Part model, mm, in its own coordinate system. A direction names the side the tool comes from. Give positions to 0.01 mm unless a question says otherwise; leave off trailing zeros. Write each loop counter-clockwise with the first axis right and the second up, starting at its lowest first coordinate (ties: lowest second). Pieces come first, ordered by that corner, then holes. Notation, with made-up numbers: M -9,41.5 L 3,41.5 A16 cw 3,69.5 Z; hole C 6.5,74 d11. An arc over 180 degrees is marked long. Write item = value, one per line. Start each with the question number.
from build123d import *

# Parameters (mm, degrees)
SKETCH1_R                                       = 3.302
BOSS_EXTRUDE1_DEPTH                             = 6.35
SKETCH2_R                                       = 16.4211
BOSS_EXTRUDE3_DEPTH                             = 6.35
BOSS_EXTRUDE3_DEPTH_BACK                        = 3.175
F_6_CLEARANCE_HOLE1_D                           = 4.3053
F_6_CLEARANCE_HOLE1_DEPTH                       = 9.525
F_6_PLASTIC_INSERT_AT_2_COUNT                   = 2
F_6_PLASTIC_INSERT_AT_2_PITCH                   = 46.355
BOSS_EXTRUDE4_REACH                             = 14.7
SKETCH22_R                                      = 16.4211
SKETCH22_R_2                                    = 3.302
CBORE_FOR_0_PAN_HEAD_MACHINE_SCREW1_D           = 1.8542
CBORE_FOR_0_PAN_HEAD_MACHINE_SCREW1_CBORE_D     = 3.57124
CBORE_FOR_0_PAN_HEAD_MACHINE_SCREW1_CBORE_DEPTH = 6.35


with BuildPart() as part:
    # Sketch1 → Boss-Extrude1 (new body)
    with BuildSketch(Plane.XY):
        with BuildLine():
            ThreePointArc((16.170566439, -2.8575), (16.4211, 0), (16.170566439, 2.8575))
            ThreePointArc((16.170566439, 2.8575), (0, 16.4211), (-16.170566439, 2.8575))
            ThreePointArc((-16.170566439, 2.8575), (-16.4211, 0), (-16.170566439, -2.8575))
            ThreePointArc((-16.170566439, -2.8575), (0, -16.4211), (16.170566439, -2.8575))
        make_face()
        Circle(SKETCH1_R, mode=Mode.SUBTRACT)
    extrude(amount=BOSS_EXTRUDE1_DEPTH)

    # Sketch2 → Boss-Extrude3 (add, two sides)
    with BuildSketch(Plane.XY.offset(6.35)) as boss_extrude3_sk:
        with BuildLine():
            Line((23.1775, 4.1275), (23.138323054, 4.1275))
            ThreePointArc((23.138323054, 4.1275), (19.696705066, 5.14104372), (17.35374229, 7.858125))
            ThreePointArc((17.35374229, 7.858125), (0, 19.05), (-17.35374229, 7.858125))
            ThreePointArc((-17.35374229, 7.858125), (-19.696705066, 5.14104372), (-23.138323054, 4.1275))
            Line((-23.138323054, 4.1275), (-23.1775, 4.1275))
            ThreePointArc((-23.1775, 4.1275), (-27.305, 0), (-23.1775, -4.1275))
            Line((-23.1775, -4.1275), (-23.138323054, -4.1275))
            ThreePointArc((-23.138323054, -4.1275), (-19.696705066, -5.14104372), (-17.35374229, -7.858125))
            ThreePointArc((-17.35374229, -7.858125), (0, -19.05), (17.35374229, -7.858125))
            ThreePointArc((17.35374229, -7.858125), (19.696705066, -5.14104372), (23.138323054, -4.1275))
            Line((23.138323054, -4.1275), (23.1775, -4.1275))
            ThreePointArc((23.1775, -4.1275), (27.305, 0), (23.1775, 4.1275))
        make_face()
        Circle(SKETCH2_R, mode=Mode.SUBTRACT)
    extrude(amount=BOSS_EXTRUDE3_DEPTH)
    extrude(boss_extrude3_sk.sketch, amount=-BOSS_EXTRUDE3_DEPTH_BACK)

    # #6 Clearance Hole1
    with Locations(Plane(origin=(-22.699598292, 0.104385938, 3.175), x_dir=(-1, 0, 0), z_dir=(0, 0, -1))):
        with Locations((-45.877098292, -0.104385938), (0.477901708, -0.104385938)):
            Hole(F_6_CLEARANCE_HOLE1_D / 2, depth=F_6_CLEARANCE_HOLE1_DEPTH)

    # Sketch5 → #6 Plastic Insert (revolve, cut)
    with BuildSketch(Plane(origin=(23.1775, 0, 3.175), x_dir=(0, 1, 0), z_dir=(1, 0, 0))):
        Polygon((0, 0), (0, 3.81), (2.5273, 3.81), (2.6543, 0), align=None)
    f_6_plastic_insert = revolve(axis=Axis((23.1775, 0, 113.175), (0, 0, -1)), mode=Mode.SUBTRACT)

    # #6 Plastic Insert at 2: #6 Plastic Insert ×2
    with Locations(*[(-i * F_6_PLASTIC_INSERT_AT_2_PITCH, 0, 0) for i in range(1, F_6_PLASTIC_INSERT_AT_2_COUNT)]):
        add(f_6_plastic_insert, mode=Mode.SUBTRACT)

    # Sketch22 → Boss-Extrude4 (add, up to next)
    with BuildSketch(Plane.XY.offset(12.7), mode=Mode.PRIVATE) as boss_extrude4_sk1:
        Circle(SKETCH22_R)
        Circle(SKETCH22_R_2, mode=Mode.SUBTRACT)
    boss_extrude4_tool1 = extrude(boss_extrude4_sk1.sketch, amount=-BOSS_EXTRUDE4_REACH, mode=Mode.PRIVATE) - part.part
    add(boss_extrude4_tool1.solids().sort_by_distance((-15.956641, 0, 12.7))[0])

    # CBORE for #0 Pan Head Machine Screw1 (through all)
    with Locations(Plane(origin=(0, 0, 0), x_dir=(-1, 0, 0), z_dir=(0, 0, -1))):
        with Locations((-7.435045578, 14.69458661), (7.747421379, 14.69458661), (7.747421379, -14.69458661), (-7.435045578, -14.69458661)):
            CounterBoreHole(CBORE_FOR_0_PAN_HEAD_MACHINE_SCREW1_D / 2, CBORE_FOR_0_PAN_HEAD_MACHINE_SCREW1_CBORE_D / 2, CBORE_FOR_0_PAN_HEAD_MACHINE_SCREW1_CBORE_DEPTH)


solid = part.part
Q1. Two-plate mould, pull along X, no slides. Class faces 1 (the face through (-27.304, 0.091, 8.004)), 2 (the face through (21.027, 0.095, 9.883)), 3 (the face through (0, 4, 0)), 4 (the face through (-0.306, -19.048, 8.004)): +X half, -X half, draft (parallel to the pull), parting line (faces both ways), or undercut.
Q2. Slice it at B-B (x = 0). Give the cut face in (y, z) (3 decimals).
Q3. Slice it at C-C (z = 10.75). Give the number of separate pieces and of enclosed holes in the cut face, and give its area (3 significant figures).
Q4. Slice it at A-A (y = 0). Give the cut face in (x, z) (3 decimals), and give its area (3 significant figures).
Q5. Probe line 1 along Y through (x, z) = (7.5, 5.75); line 2 along X through (y, z) = (0.5, 4.75); line 3 along Y through (x, z) = (-1.5, 8.75). List the from-to ranges inside material, lowest first.
Q6. Drop flat-ended pins along their axis: P1, Ø1, axis at x = -5, z = 1.5, coming from the +Y side; P2, Ø6, axis at x = -11.5, z = 8, coming from the -Y side; P3, Ø1, axis at y = -3.5, z = 7, coming from the +X side. Give the stop position or say it passes through.
Q7. Tool access for faces 5 (the face through (-22, -2, 6.985)), 6 (the face through (-0.23, -16.42, 1.57)), 7 (the face through (-0.06, 16.42, 1.57)): list every direction of +Z, -Z, +X, -X, +Y, -Y with a clear straight run to the whole face (end or side of a thin tool).
Working result:
q1.face_1 = -X half
q1.face_2 = undercut
q1.face_3 = draft
q1.face_4 = parting line
q2.outline = M -19.05,3.175 L -16.421,3.175 L -16.421,0 L -3.302,0 L -3.302,12.7 L -19.05,12.7 Z; M 3.302,0 L 16.421,0 L 16.421,3.175 L 19.05,3.175 L 19.05,12.7 L 3.302,12.7 Z
q3.separate_pieces = 1
q3.enclosed_holes = 7
q3.area = 1,200 mm2
q4.outline = M -27.305,3.175 L -25.832,3.175 L -25.705,6.985 L -25.33,6.985 L -25.33,12.7 L -27.305,12.7 Z; M -21.025,6.985 L -20.65,6.985 L -20.523,3.175 L -16.421,3.175 L -16.421,0 L -3.302,0 L -3.302,12.7 L -21.025,12.7 Z; M 3.302,0 L 16.421,0 L 16.421,3.175 L 20.523,3.175 L 20.65,6.985 L 21.025,6.985 L 21.025,12.7 L 3.302,12.7 Z; M 25.33,6.985 L 25.705,6.985 L 25.832,3.175 L 27.305,3.175 L 27.305,12.7 L 25.33,12.7 Z
q4.area = 452 mm2
q5.line_1 = -17.51 to -16.48, -12.91 to 12.91, 16.48 to 17.51
q5.line_2 = -27.27 to -25.73, -20.62 to -3.26, 3.26 to 20.62, 25.73 to 27.27
q5.line_3 = -18.99 to -2.94, 2.94 to 18.99
q6.P1 = 15.79
q6.P2 = -17.05
q6.P3 = 26.01
q7.face_5 = -Z
q7.face_6 = -Z, -Y
q7.face_7 = -Z, +Y
